from build123d import *

# Parameters (mm, degrees)
SKETCH1_W           = 254
SKETCH1_H           = 254
BOSS_EXTRUDE1_DEPTH = 5.08
SKETCH2_R           = 2.10058
CUT_EXTRUDE1_DEPTH  = 6.08
SKETCH5_R           = 4.399999963
CUT_EXTRUDE2_DEPTH  = 6.08


with BuildPart() as part:
    # Sketch1 → Boss-Extrude1 (new body)
    with BuildSketch(Plane(origin=(0, 0, 0), x_dir=(1, 0, 0), z_dir=(0, 1, 0))):
        Rectangle(SKETCH1_W, SKETCH1_H)
    extrude(amount=BOSS_EXTRUDE1_DEPTH)

    # Sketch2 → Cut-Extrude1 (cut, through all)
    with BuildSketch(Plane(origin=(0, 5.08, 0), x_dir=(1, 0, 0), z_dir=(0, 1, 0))):
        with Locations((0, 15.499969)):
            Circle(SKETCH2_R)
        with Locations((13.423366912, -7.7499845)):
            Circle(SKETCH2_R)
        with Locations((-13.423366912, -7.7499845)):
            Circle(SKETCH2_R)
    extrude(amount=-CUT_EXTRUDE1_DEPTH, mode=Mode.SUBTRACT)

    # Sketch5 → Cut-Extrude2 (cut, through all)
    with BuildSketch(Plane(origin=(0, 5.08, 0), x_dir=(1, 0, 0), z_dir=(0, 1, 0))):
        with Locations((66.542698013, 66.4572719)):
            Circle(SKETCH5_R)
        with Locations((66.542698013, -66.542698013)):
            Circle(SKETCH5_R)
        with Locations((-66.4572719, -66.542698013)):
            Circle(SKETCH5_R)
        with Locations((-66.4572719, 66.4572719)):
            Circle(SKETCH5_R)
    extrude(amount=-CUT_EXTRUDE2_DEPTH, mode=Mode.SUBTRACT)


solid = part.part
Check sheet for the modelled part. Datum: model origin and axes. Units: mm. Round coordinates to 2 decimals unless told otherwise and drop trailing zeros. One line per item, written item: value.
(1) Release check for a two-part mould opening along X. For faces 1 (the face through (65.59, 2.58, -62.16)), 2 (the face through (65.59, 2.58, 70.84)), 3 (the face through (-2, 5.08, -2)) record: +X half, -X half, draft (parallel to the pull), parting line (faces both ways), or undercut.
Computed values:
face 1: undercut
face 2: undercut
face 3: draft
(2) Depth check by flat-ended pin: pin 1 Ø5.5 at (x, z) = (0, -15.5) entering from -Y. Enter the tip coordinate at first touch or a pass-through.
Computed values:
pin 1: stops at y = 0
(3) Thickness scan on line 1 (X direction, y = 1.4, z = -67); line 2 (Z direction, x = 0, y = 1.2); line 3 (Z direction, x = -12.5, y = 4.4). Record the ranges inside material, lowest first.
Computed values:
line 1: x = -127 to -70.82, -62.09 to 62.18, 70.91 to 127
line 2: z = -127 to -17.6, -13.4 to 127
line 3: z = -127 to 5.86, 9.64 to 127
